Input: part model. Units: mm. Frame: model coordinates. A direction names the side the tool comes from. Coordinates: 2 decimals unless noted, no trailing zeros. Loops run counter-clockwise (first coordinate to the right, second up) from the corner with the lowest first, then second, coordinate; pieces in that order, holes last.
Item 1: Section B-B on z = 1.5. Return loops of the section in (x, y).
Item 2: Section A-A on y = -2.6. Return loops of the section in (x, z), and give its area (3 significant figures).
Item 3: Contact query for flat-ended pins moving along their axis: P1, Ø3.5, axis at x = 0, y = -7.5, coming from the -Z side; P2, Ø0.5, axis at y = -6.5, z = -1, coming from the +X side; P3, Ø1.8, axis at x = 0, y = -7.7, coming from the +Z side. Output: stop coordinate, or through.
Item 4: Section C-C on z = 4.8. Return loops of the section in (x, y).
Item 5: Ray query, line 1 along Y through (x, z) = (1.5, -4.8); line 2 along Y through (x, z) = (0, 8.1); line 3 along Y through (x, z) = (0, -8.1). Return the intervals inside material, ascending.
Item 6: Section D-D on x = 0. Give the number of separate pieces and of enclosed holes in the cut face, and give its area (3 significant figures).
Item 7: Pull-direction query (Z, two-part tool) for faces 6 (the cylindrical face through (-0.104, -6.907, -0.831)), 7 (the flat face through (0, -5.1, -7.5)), 8 (the flat face through (0, -5.6, -5)), 9 (the flat face through (0, 0, -9.9)); classes: released by +Z, released by -Z, zero draft, split by the parting line, or undercut.
Item 8: Reachability of faces 1 (the flat face through (1.85, 6, 3)), 2 (the flat face through (0.4, -6.8, -8.435)), 3 (the cylindrical face through (-0.05, 4.17, -9.66)), 4 (the cylindrical face through (0.05, -4.86, 9.67)), 5 (the flat face through (-0.4, -6.8, -0.535)) from +Z, -Z, +X, -X, +Y, -Y: full face, straight path, thin tool, end or side. Return the list, or none.
```python
from build123d import *

# Parameters (mm, degrees)
SKETCH_1_R          = 1.25
EXTRUDE_1_DEPTH     = 3.25
SKETCH_4_W          = 0.6
SKETCH_4_H          = 4.2
EXTRUDE_4_DEPTH     = 1.6
FILLET_1_R          = 0.8
SKETCH_2_W          = 3.7
SKETCH_2_H          = 1.9
EXTRUDE_2_DEPTH     = 1.3
FILLET_2_R          = 0.8
EXTRUDE_3_DEPTH     = 2
FILLET_4_R          = 0.2
FILLET_3_R          = 0.4
SKETCH_5_R          = 0.8
CUT_EXTRUDE_1_DEPTH = 16.7


with BuildPart() as part:
    # Эскиз1 → Бобышка-Вытянуть1 (new body, symmetric)
    with BuildSketch(Plane(origin=(0, 0, 0), x_dir=(0, 0, -1), z_dir=(1, 0, 0))):
        Polygon((-9.9, 5.1), (-9.9, -5.1), (-6.9, -5.1), (-6.4, -5.6), (-3.2, -5.6), (-2.7, -5.1), (2.7, -5.1), (3.2, -5.6), (6.4, -5.6), (6.9, -5.1), (9.9, -5.1), (9.9, 4.4), (0.3, 4.4), (-0.4, 5.1), align=None)
        with Locations((-4.8, -2.6)):
            Circle(SKETCH_1_R, mode=Mode.SUBTRACT)
        with Locations((4.8, -2.6)):
            Circle(SKETCH_1_R, mode=Mode.SUBTRACT)
    extrude(amount=EXTRUDE_1_DEPTH, both=True)

    # Эскиз4 → Бобышка-Вытянуть4 (add, symmetric)
    with BuildSketch(Plane(origin=(0, 0, 0), x_dir=(0, 0, -1), z_dir=(1, 0, 0))):
        with Locations((0.834899724, -7.2)):
            Rectangle(SKETCH_4_W, SKETCH_4_H)
        with Locations((-7.965100276, -7.2)):
            Rectangle(SKETCH_4_W, SKETCH_4_H)
        with Locations((8.134899724, -7.2)):
            Rectangle(SKETCH_4_W, SKETCH_4_H)
    extrude(amount=EXTRUDE_4_DEPTH, both=True)

    # Скругление1
    fillet_1_edges = [part.edges().sort_by_distance(p)[0] for p in [
        (0, -5.1, 9.9),
        (0, 5.1, 9.9),
        (0, 4.4, -9.9),
        (0, -5.1, -9.9),
        (-1.6, -9.3, 7.965100276),
        (1.6, -9.3, 7.965100276),
        (-1.6, -9.3, -0.834899724),
        (1.6, -9.3, -0.834899724),
        (-1.6, -9.3, -8.134899724),
        (1.6, -9.3, -8.134899724),
    ]]
    fillet(fillet_1_edges, radius=FILLET_1_R)

    # Эскиз2 → Бобышка-Вытянуть2 (add)
    with BuildSketch(Plane(origin=(0, 5.1, 0), x_dir=(1, 0, 0), z_dir=(0, 1, 0))):
        with Locations((0, -2.75)):
            Rectangle(SKETCH_2_W, SKETCH_2_H)
    extrude(amount=EXTRUDE_2_DEPTH)

    # Скругление2
    fillet_2_edges = [part.edges().sort_by_distance(p)[0] for p in [
        (0, 6.4, 1.8),
        (0, 6.4, 3.7),
    ]]
    fillet(fillet_2_edges, radius=FILLET_2_R)

    # Эскиз3 → Бобышка-Вытянуть3 (add, symmetric)
    with BuildSketch(Plane(origin=(0, 0, 0), x_dir=(0, 0, -1), z_dir=(1, 0, 0))):
        with BuildLine():
            Line((-6.9, 5.1), (-6.9, 5.7))
            Line((-6.9, 5.7), (8.447548782, 10.22247127))
            ThreePointArc((8.447548782, 10.22247127), (10.327160868, 12.885134856), (13.241910115, 11.426726206))
            Line((13.241910115, 11.426726206), (13.048790165, 11.369819437))
            ThreePointArc((13.048790165, 11.369819437), (10.286090587, 12.666664311), (8.668057439, 10.078946335))
            Line((8.668057439, 10.078946335), (-6.7, 5.550431767))
            Line((-6.7, 5.550431767), (-6.7, 5.1))
            Line((-6.7, 5.1), (-6.9, 5.1))
        make_face()
    extrude(amount=EXTRUDE_3_DEPTH, both=True)

    # Скругление4
    fillet_4_edges = [part.edges().sort_by_distance(p)[0] for p in [
        (0, 5.550431767, 6.7),
        (0, 10.22247127, -8.447548782),
    ]]
    fillet(fillet_4_edges, radius=FILLET_4_R)

    # Скругление3
    fillet_3_edges = [part.edges().sort_by_distance(p)[0] for p in [
        (0, 10.078946335, -8.668057439),
        (0, 5.7, 6.9),
    ]]
    fillet(fillet_3_edges, radius=FILLET_3_R)

    # Эскиз5 → Вырез-Вытянуть1 (cut)
    with BuildSketch(Plane.XY.offset(8.265100276)):
        with Locations((0, -7.7)):
            Circle(SKETCH_5_R)
    extrude(amount=-CUT_EXTRUDE_1_DEPTH, mode=Mode.SUBTRACT)


solid = part.part
```
Results found:
1. outline: (-3.25, -5.1) - (3.25, -5.1) - (3.25, 5.1) - (-3.25, 5.1) - close; (-2, 7.08) - (2, 7.08) - (2, 7.29) - (-2, 7.29) - close
2. outline: (-3.25, -9.9) - (3.25, -9.9) - (3.25, -6.05) - (-3.25, -6.05) - close; (-3.25, -3.55) - (3.25, -3.55) - (3.25, 3.55) - (-3.25, 3.55) - close; (-3.25, 6.05) - (3.25, 6.05) - (3.25, 9.9) - (-3.25, 9.9) - close
2. area: 96.2 mm2
3. P1: stops at z = -8.43
3. P2: stops at x = 1.6
3. P3: stops at z = 8.27
4. outline: (-3.25, -5.6) - (3.25, -5.6) - (3.25, -3.85) - (-3.25, -3.85) - close; (-3.25, -1.35) - (3.25, -1.35) - (3.25, 5.1) - (-3.25, 5.1) - close; (-2, 6.11) - (2, 6.11) - (2, 6.32) - (-2, 6.32) - close
5. line 1: y = -5.6 to -3.85, -1.35 to 4.4, 8.94 to 9.15
5. line 2: y = -9.3 to -8.5, -6.9 to 5.1
5. line 3: y = -9.3 to -8.5, -6.9 to 4.4, 9.91 to 10.12
6. separate pieces: 4
6. enclosed holes: 2
6. area: 200 mm2
7. face 6: zero draft
7. face 7: undercut
7. face 8: undercut
7. face 9: released by -Z
8. face 1: -Z, +X
8. face 2: -Z, +X, -X, -Y
8. face 3: -Z, +X, -X
8. face 4: +Z, +X, -X, -Y
8. face 5: +X, -X, -Y
